Drawing for the job (mm, zero at the part's lowest x, y, z). A direction names the side the tool comes from. Round coordinates to 2 decimals unless told otherwise and drop trailing zeros. Write each loop counter-clockwise with the first axis right and the second up, starting at its lowest first coordinate (ties: lowest second). Pieces come first, ordered by that corner, then holes. Notation, with made-up numbers: M -23,82.25 L 13,82.25 A21 ccw 13,100.25 Z; hole C 69.25,20 d3. An arc over 180 degrees is marked long. Use a Markdown table: item, result. Add a question column.
1) Which spindle directions (+Z, -Z, +X, -X, +Y, -Y) get a long thin tool onto all of the face, cutting with end or side? Do the marked faces 1 and 2. Say none if no direction does.
2) Wall check: probe 1 along Z at (x, y) = (94, 66.5); probe 2 along Z at (x, y) = (28, 52); probe 3 along X at (y, z) = (73.5, 67). Give the ranges that are in metal, low to high.
3) Drop flat-ended pins along their axis: P1, Ø10, axis at x = 17.5, z = 57, coming from the -Y side; P2, Ø2.5, axis at y = 44, z = 76.5, coming from the +X side; P3, Ø1.5, axis at y = 52.5, z = 77, coming from the -X side; P4, Ø1.5, axis at x = 61, y = 24.5, coming from the +Z side. Give the stop position or say it passes through.
4) Slice it at B-B on x = 70.5. Write the cut outline in (y, z).
5) Slice it at A-A on y = 50. Write the cut outline in (x, z).
6) Slice it at D-D on x = 16.5. Write the cut outline in (y, z).
7) Slice it at C-C on z = 69. Write the cut outline in (x, y).
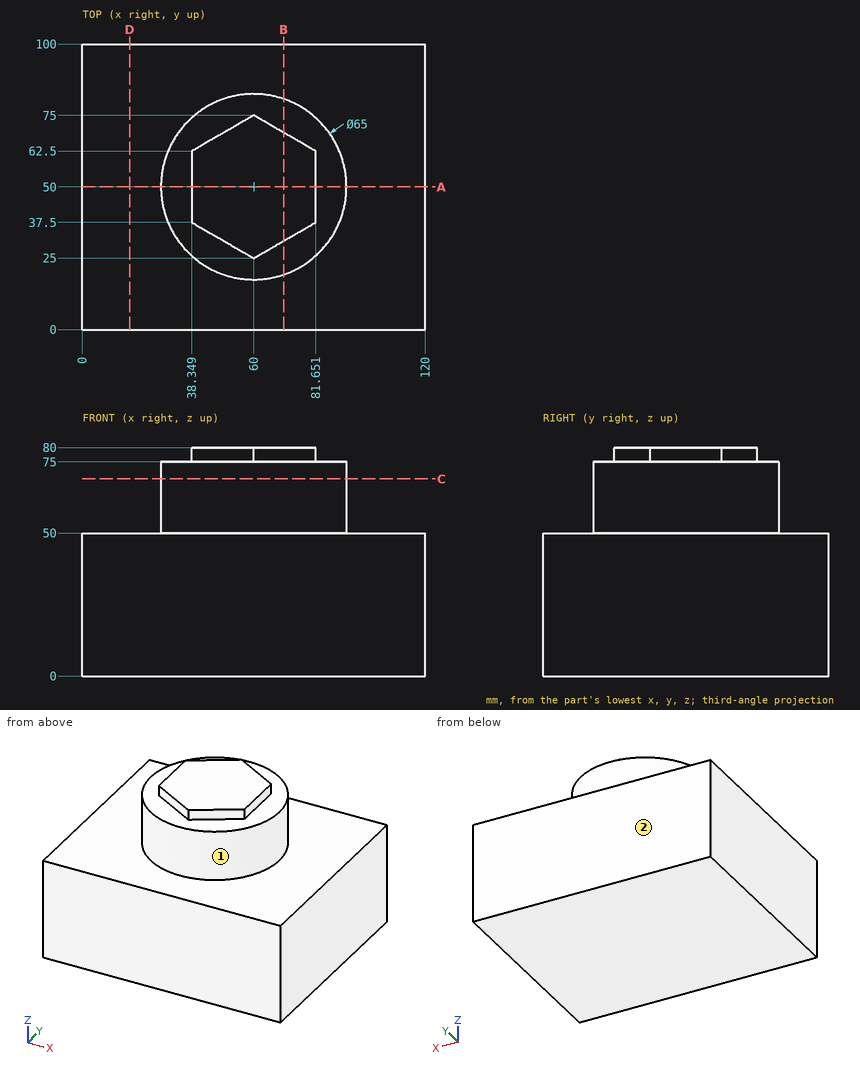
Entries:
| question | item | result |
|---|---|---|
| 1 | face 1 | +Z |
| 1 | face 2 | +Z, -Z, +X, -X, +Y |
| 2 | probe 1 | z = 0 to 50 |
| 2 | probe 2 | z = 0 to 75 |
| 2 | probe 3 | x = 37.55 to 82.45 |
| 3 | P1 | passes through |
| 3 | P2 | stops at x = 81.65 |
| 3 | P3 | stops at x = 38.35 |
| 3 | P4 | stops at z = 75 |
| 4 | outline | M 0,0 L 100,0 L 100,50 L 80.76,50 L 80.76,75 L 68.94,75 L 68.94,80 L 31.06,80 L 31.06,75 L 19.24,75 L 19.24,50 L 0,50 Z |
| 5 | outline | M 0,0 L 120,0 L 120,50 L 92.5,50 L 92.5,75 L 81.65,75 L 81.65,80 L 38.35,80 L 38.35,75 L 27.5,75 L 27.5,50 L 0,50 Z |
| 6 | outline | M 0,0 L 100,0 L 100,50 L 0,50 Z |
| 7 | outline | C 60,50 d65 |
